Answer from the drawing. Dimensions are ordinates in mm from the lowest x, y and z of the part. Coordinates: 2 decimals unless noted, no trailing zeros. Order: outer loops, then holes, each group sorted by start corner. A loop starts at its lowest first (then second) coordinate and runs counter-clockwise, first axis right, second up. Notation, with made-up numbers: (79.25, 59.5) -> (136.25, 59.5) arc R7 cw to (136.25, 63.5) -> close; hole circle Ø8 at (-7, -16.5). An arc over 180 degrees is marked (long way). Answer in a Markdown table with one row per item.
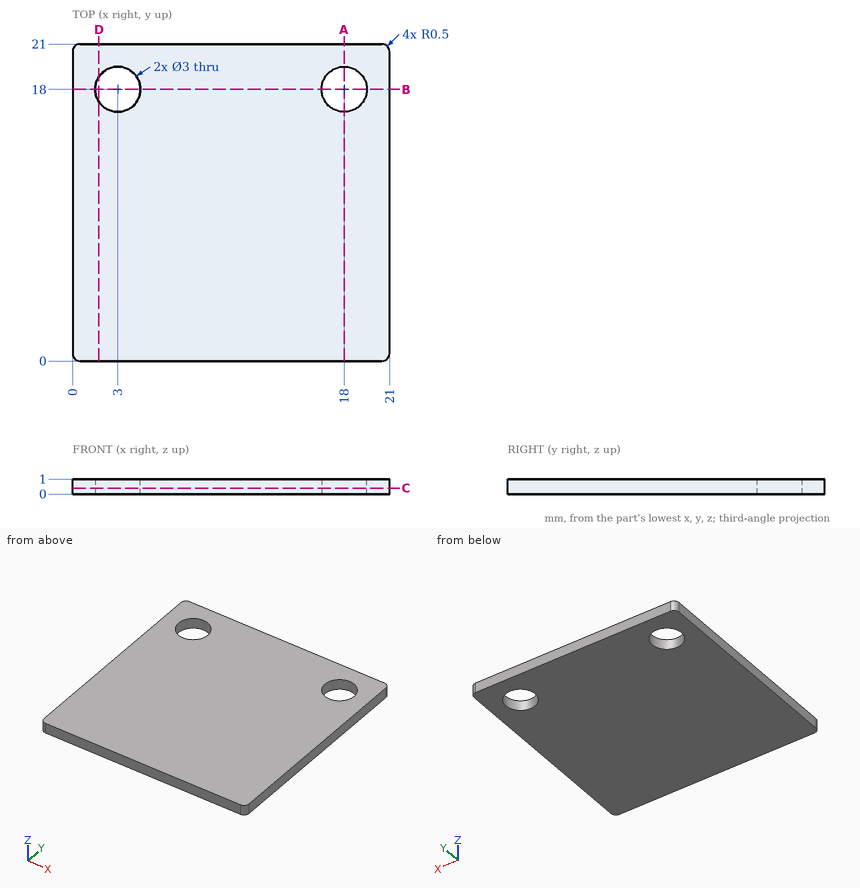
Q1. The part is cut by section B-B (y = 18). Write down the section's boundary in (x, z), then the cut area to 3 significant figures.
Outcome:
| item | result |
|---|---|
| outline | (0, 0) -> (1.5, 0) -> (1.5, 1) -> (0, 1) -> close; (4.5, 0) -> (16.5, 0) -> (16.5, 1) -> (4.5, 1) -> close; (19.5, 0) -> (21, 0) -> (21, 1) -> (19.5, 1) -> close |
| area | 15.0 mm² |
Q2. Given pin 1 (2.5 mm diameter, centred on x = 3, y = 18, fed in from -Z), flat-ended and moving along its own axis, determine where the tip first touches the part or whether it passes through.
Outcome:
| item | result |
|---|---|
| pin 1 | through |
Q3. The part is cut by section D-D (x = 1.75). Write down the section's boundary in (y, z), then the cut area to 3 significant figures.
Outcome:
| item | result |
|---|---|
| outline | (0, 0) -> (17.17, 0) -> (17.17, 1) -> (0, 1) -> close; (18.83, 0) -> (21, 0) -> (21, 1) -> (18.83, 1) -> close |
| area | 19.3 mm² |
Q4. The part is cut by section A-A (x = 18). Write down the section's boundary in (y, z).
Outcome:
| item | result |
|---|---|
| outline | (0, 0) -> (16.5, 0) -> (16.5, 1) -> (0, 1) -> close; (19.5, 0) -> (21, 0) -> (21, 1) -> (19.5, 1) -> close |
Q5. The part is cut by section C-C (z = 0.4). Write down the section's boundary in (x, y).
Outcome:
| item | result |
|---|---|
| outline | (0, 0.5) arc R0.5 ccw to (0.5, 0) -> (20.5, 0) arc R0.5 ccw to (21, 0.5) -> (21, 20.5) arc R0.5 ccw to (20.5, 21) -> (0.5, 21) arc R0.5 ccw to (0, 20.5) -> close; hole circle Ø3 at (3, 18); hole circle Ø3 at (18, 18) |
Q6. Consider line 1 (X direction, y = 18, z = 0.65); line 2 (X direction, y = 19.25, z = 0.8); line 3 (Y direction, x = 3, z = 0.6). Determine where each line is inside the solid, lowest interval first.
Outcome:
| item | result |
|---|---|
| line 1 | 0 to 1.5, 4.5 to 16.5, 19.5 to 21 |
| line 2 | 0 to 2.17, 3.83 to 17.17, 18.83 to 21 |
| line 3 | 0 to 16.5, 19.5 to 21 |
